Read the model definition and answer for the solid it produces. Units are mm, in the model's axes. A direction names the side the tool comes from. Coordinates: 2 decimals unless noted, no trailing zeros. Order: outer loops, then holes, each group sorted by start corner. A loop starts at its lowest first (then second) coordinate and runs counter-clockwise, first axis right, second up. Notation, with made-up numbers: M -7.75,-2 L 0.25,-2 A15 ccw 0.25,9 Z; hole C 14,17.25 d11. An arc over 180 degrees is marked long. One line per question, with ' | ' between items. Start each with the question number.
1) Find section B-B, the plane y = 0.75. Write down the section's boundary in (x, z).
2) Find section C-C, the plane z = -41.5. Write down the section's boundary in (x, y), plus the area to 3 significant figures.
3) Find section D-D, the plane z = -50. Write down the section's boundary in (x, y).
4) The mould has two halves that part along X. Classify faces 4 (the face through (57.54, 0.69, -21)), 5 (the face through (56.076, 0.689, -61.197)), 6 (the face through (52.21, 0.86, -27.73)), 7 (the face through (54, 1, -17.667)): +X half, -X half, draft (parallel to the pull), parting line (faces both ways), or undercut.
5) Consider probe 1 along Z at (x, y) = (56.75, 0.6); probe 2 along Z at (x, y) = (54.75, 0.5); probe 3 along X at (y, z) = (0.7, -59). Determine where each line is inside the solid, lowest interval first.
6) A tool of negligible diameter and unlimited length cuts with its end or side. For faces 1 (the face through (53.9, 0.18, -34.82)), 2 (the face through (57, 0, -46)), 3 (the face through (58.252, 1, -61)), from which of +Z, -Z, +X, -X, +Y, -Y can it reach the whole face along a straight path? Write none if from no direction.
7) Given P1, Ø2.5, axis at x = 54.95, z = -59.43, coming from the +Y side, flat-ended and moving along its own axis, determine where the tip first touches the part or whether it passes through.
8) Find section A-A, the plane x = 54.75. Write down the section's boundary in (y, z), plus the area to 3 significant figures.
from build123d import *

# Parameters (mm, degrees)
SKETCH1_R           = 2.0955
BOSS_EXTRUDE1_DEPTH = 1.397
CUT_EXTRUDE1_DEPTH  = 52.451
FILLET1_R           = 0.762


with BuildPart() as part:
    # Sketch1 → Boss-Extrude1 (new body)
    with BuildSketch(Plane(origin=(0, 0, 0), x_dir=(1, 0, 0), z_dir=(0, 1, 0))):
        with BuildLine():
            Line((58.251832272, 62.407600024), (58.251832272, 58.66827713))
            Line((58.251832272, 58.66827713), (60.283832272, 58.66827713))
            Line((60.283832272, 58.66827713), (60.283832272, 27.93427713))
            ThreePointArc((60.283832272, 27.93427713), (60.006877388, 25.830595931), (59.194886754, 23.87027713))
            Line((59.194886754, 23.87027713), (55.613371084, 17.666910021))
            Line((55.613371084, 17.666910021), (51.815116638, 17.666910021))
            ThreePointArc((51.815116638, 17.666910021), (52.382112404, 19.118650157), (51.757304959, 20.546462917))
            ThreePointArc((51.757304959, 20.546462917), (52.324300725, 21.998203054), (51.69949328, 23.426015814))
            ThreePointArc((51.69949328, 23.426015814), (52.266489046, 24.87775595), (51.641681601, 26.305568711))
            ThreePointArc((51.641681601, 26.305568711), (52.208677367, 27.757308847), (51.583869921, 29.185121607))
            ThreePointArc((51.583869921, 29.185121607), (52.150865688, 30.636861744), (51.526058242, 32.064674504))
            ThreePointArc((51.526058242, 32.064674504), (52.093054008, 33.51641464), (51.468246563, 34.944227401))
            ThreePointArc((51.468246563, 34.944227401), (52.035242329, 36.395967537), (51.410434884, 37.823780298))
            ThreePointArc((51.410434884, 37.823780298), (51.97743065, 39.275520434), (51.352623205, 40.703333194))
            ThreePointArc((51.352623205, 40.703333194), (51.919618971, 42.155073331), (51.294811526, 43.582886091))
            ThreePointArc((51.294811526, 43.582886091), (51.861807292, 45.034626227), (51.236999847, 46.462438988))
            ThreePointArc((51.236999847, 46.462438988), (51.803995613, 47.914179124), (51.179188167, 49.341991884))
            ThreePointArc((51.179188167, 49.341991884), (51.410778499, 50.327179124), (51.139832272, 51.30227713))
            Line((51.139832272, 51.30227713), (51.139832272, 61.721904416))
            ThreePointArc((51.139832272, 61.721904416), (54.523146654, 63.855838676), (58.251832272, 62.407600024))
        make_face()
        with Locations((54.949832272, 59.43027713)):
            Circle(SKETCH1_R, mode=Mode.SUBTRACT)
    extrude(amount=BOSS_EXTRUDE1_DEPTH)

    # Sketch2 → Cut-Extrude1 (cut)
    with BuildSketch(Plane.XY):
        Polygon((55.613371084, 0), (51.139832272, 0.470187876), (51.139832272, 0), align=None)
    extrude(amount=-CUT_EXTRUDE1_DEPTH, mode=Mode.SUBTRACT)

    # Fillet1
    fillet1_edges = [part.edges().sort_by_distance(p)[0] for p in [
        (58.251832272, 0.6985, -58.66827713),
        (60.283832272, 0.6985, -58.66827713),
        (55.613371084, 0.6985, -17.666910021),
    ]]
    fillet(fillet1_edges, radius=FILLET1_R)


solid = part.part
Report:
1) outline: M 51.14,-61.72 A4.45 ccw 58.25,-62.41 L 58.25,-59.43 A0.76 cw 59.01,-58.67 L 59.52,-58.67 A0.76 ccw 60.28,-57.91 L 60.28,-27.93 A8.13 ccw 59.19,-23.87 L 55.83,-18.05 A0.76 ccw 55.17,-17.67 L 51.82,-17.67 A2.04 cw 51.76,-20.55 A2.04 cw 51.7,-23.43 A2.04 cw 51.64,-26.31 A2.04 cw 51.58,-29.19 A2.04 cw 51.53,-32.06 A2.04 cw 51.47,-34.94 A2.04 cw 51.41,-37.82 A2.04 cw 51.35,-40.7 A2.04 cw 51.29,-43.58 A2.04 cw 51.24,-46.46 A2.04 cw 51.18,-49.34 A2.04 cw 51.14,-51.3 Z; hole C 54.95,-59.43 d4.19
2) outline: M 51.83,0.4 L 55.61,0 L 60.28,0 L 60.28,1.4 L 51.83,1.4 Z | area: 11.1 mm^2
3) outline: M 51.39,0.44 L 55.61,0 L 60.28,0 L 60.28,1.4 L 51.39,1.4 Z
4) face 4: +X half | face 5: undercut | face 6: -X half | face 7: draft
5) probe 1: z = -63.5 to -60.5, -58.36 to -19.64 | probe 2: z = -63.87 to -61.52, -57.34 to -17.67 | probe 3: x = 51.14 to 52.9, 57 to 58.38
6) face 1: +Z, -X, -Y | face 2: +Z, -Z, +X, -X, -Y | face 3: -Z, +X, +Y, -Y
7) P1: passes through
8) outline: M 0,-63.87 L 1.4,-63.87 L 1.4,-61.52 L 0,-61.52 Z; M 0,-57.34 L 1.4,-57.34 L 1.4,-17.67 L 0.09,-17.67 L 0.09,-52.45 L 0,-52.45 Z | area: 55.6 mm^2
